from build123d import *

# Parameters (mm, degrees)
BOX005_W               = 0.7
BOX005_H               = 0.7
BOX005_DEPTH           = 6
BOX006_W               = 0.7
BOX006_H               = 0.7
BOX006_DEPTH           = 6
BOX007_W               = 0.7
BOX007_H               = 0.7
BOX007_DEPTH           = 6
BOX004_W               = 0.7
BOX004_H               = 0.7
BOX004_DEPTH           = 6
BOX009_W               = 10
BOX009_H               = 26
BOX009_DEPTH           = 2.7
BOX010_W               = 8.5
BOX010_H               = 15.8
BOX010_DEPTH           = 14
FILLET001_R            = 2
BOX008_W               = 10
BOX008_H               = 26
BOX008_DEPTH           = 2.7
CYLINDER001_R          = 1.6
CYLINDER001_DEPTH      = 8
CYLINDER002_R          = 1.6
CYLINDER002_DEPTH      = 8
CYLINDER003_R          = 1.6
CYLINDER003_DEPTH      = 8
CYLINDER004_R          = 1.6
CYLINDER004_DEPTH      = 8
CYLINDER005_R          = 1.6
CYLINDER005_DEPTH      = 8
CYLINDER006_R          = 1.6
CYLINDER006_DEPTH      = 8
CYLINDER007_R          = 1.6
CYLINDER007_DEPTH      = 8
CYLINDER_R             = 1.6
CYLINDER_DEPTH         = 8
BOX003_W               = 10
BOX003_H               = 10
BOX003_DEPTH           = 10
BOX003_ROLL_ANGLE      = 40.999967
BOX003_PLACEMENT_ANGLE = 180
BOX002_W               = 10
BOX002_H               = 10
BOX002_DEPTH           = 10
BOX002_ROLL_ANGLE      = 40.999967
BOX001_W               = 9.7
BOX001_H               = 17
BOX001_DEPTH           = 20.299999
FILLET_R               = 2


with BuildPart() as pin001:
    # Box005 → Box005 (new body)
    with BuildSketch(Plane(origin=(-5.35, 7.15, -3), x_dir=(1, 0, 0), z_dir=(0, 0, 1))):
        with Locations((0.35, 0.35)):
            Rectangle(BOX005_W, BOX005_H)
    extrude(amount=BOX005_DEPTH)


with BuildPart() as pin002:
    # Box006 → Box006 (new body)
    with BuildSketch(Plane(origin=(-5.35, -7.85, -3), x_dir=(1, 0, 0), z_dir=(0, 0, 1))):
        with Locations((0.35, 0.35)):
            Rectangle(BOX006_W, BOX006_H)
    extrude(amount=BOX006_DEPTH)


with BuildPart() as pin003:
    # Box007 → Box007 (new body)
    with BuildSketch(Plane(origin=(4.65, -7.85, -3), x_dir=(1, 0, 0), z_dir=(0, 0, 1))):
        with Locations((0.35, 0.35)):
            Rectangle(BOX007_W, BOX007_H)
    extrude(amount=BOX007_DEPTH)


with BuildPart() as pins:
    # Box004 → Box004 (new body)
    with BuildSketch(Plane(origin=(4.65, 7.15, -3), x_dir=(1, 0, 0), z_dir=(0, 0, 1))):
        with Locations((0.35, 0.35)):
            Rectangle(BOX004_W, BOX004_H)
    extrude(amount=BOX004_DEPTH)

    # Fusion003: union Pin001, Pin002, Pin003
    add(pin001.part)
    add(pin002.part)
    add(pin003.part)


with BuildPart() as box009:
    # Box009 → Box009 (new body)
    with BuildSketch(Plane(origin=(-2.25, 13, 0), x_dir=(-1, 0, 0), z_dir=(0, 0, 1))):
        with Locations((5, 13)):
            Rectangle(BOX009_W, BOX009_H)
    extrude(amount=BOX009_DEPTH)


with BuildPart() as fillet001:
    # Box010 → Box010 (new body)
    with BuildSketch(Plane(origin=(-4.25, -7.9, 0), x_dir=(1, 0, 0), z_dir=(0, 0, 1))):
        with Locations((4.25, 7.9)):
            Rectangle(BOX010_W, BOX010_H)
    extrude(amount=BOX010_DEPTH)

    # Fillet001
    fillet001_edges = [fillet001.edges().sort_by_distance(p)[0] for p in [
        (-4.25, -7.9, 7),
        (-4.25, 7.9, 7),
        (4.25, -7.9, 7),
        (4.25, 7.9, 7),
    ]]
    fillet(fillet001_edges, radius=FILLET001_R)


with BuildPart() as fusion004:
    # Box008 → Box008 (new body)
    with BuildSketch(Plane(origin=(2.25, -13, 0), x_dir=(1, 0, 0), z_dir=(0, 0, 1))):
        with Locations((5, 13)):
            Rectangle(BOX008_W, BOX008_H)
    extrude(amount=BOX008_DEPTH)

    # Fusion004: union Box009, Fillet001
    add(box009.part)
    add(fillet001.part)


with BuildPart() as cylinder001:
    # Cylinder001 → Cylinder001 (new body)
    with BuildSketch(Plane(origin=(-5, 2.5, 0), x_dir=(1, 0, 0), z_dir=(0, 0, 1))):
        Circle(CYLINDER001_R)
    extrude(amount=CYLINDER001_DEPTH)


with BuildPart() as cylinder002:
    # Cylinder002 → Cylinder002 (new body)
    with BuildSketch(Plane(origin=(-5, -2.5, 0), x_dir=(1, 0, 0), z_dir=(0, 0, 1))):
        Circle(CYLINDER002_R)
    extrude(amount=CYLINDER002_DEPTH)


with BuildPart() as cylinder003:
    # Cylinder003 → Cylinder003 (new body)
    with BuildSketch(Plane(origin=(-5, -7.5, 0), x_dir=(1, 0, 0), z_dir=(0, 0, 1))):
        Circle(CYLINDER003_R)
    extrude(amount=CYLINDER003_DEPTH)


with BuildPart() as cylinder004:
    # Cylinder004 → Cylinder004 (new body)
    with BuildSketch(Plane(origin=(5, 7.5, 0), x_dir=(1, 0, 0), z_dir=(0, 0, 1))):
        Circle(CYLINDER004_R)
    extrude(amount=CYLINDER004_DEPTH)


with BuildPart() as cylinder005:
    # Cylinder005 → Cylinder005 (new body)
    with BuildSketch(Plane(origin=(5, 2.5, 0), x_dir=(1, 0, 0), z_dir=(0, 0, 1))):
        Circle(CYLINDER005_R)
    extrude(amount=CYLINDER005_DEPTH)


with BuildPart() as cylinder006:
    # Cylinder006 → Cylinder006 (new body)
    with BuildSketch(Plane(origin=(5, -2.5, 0), x_dir=(1, 0, 0), z_dir=(0, 0, 1))):
        Circle(CYLINDER006_R)
    extrude(amount=CYLINDER006_DEPTH)


with BuildPart() as cylinder007:
    # Cylinder007 → Cylinder007 (new body)
    with BuildSketch(Plane(origin=(5, -7.5, 0), x_dir=(1, 0, 0), z_dir=(0, 0, 1))):
        Circle(CYLINDER007_R)
    extrude(amount=CYLINDER007_DEPTH)


with BuildPart() as pinholder:
    # Cylinder → Cylinder (new body)
    with BuildSketch(Plane(origin=(-5, 7.5, 0), x_dir=(1, 0, 0), z_dir=(0, 0, 1))):
        Circle(CYLINDER_R)
    extrude(amount=CYLINDER_DEPTH)

    # Fusion001: union Cylinder001, Cylinder002, Cylinder003, Cylinder004, Cylinder005, Cylinder006, Cylinder007
    add(cylinder001.part)
    add(cylinder002.part)
    add(cylinder003.part)
    add(cylinder004.part)
    add(cylinder005.part)
    add(cylinder006.part)
    add(cylinder007.part)


with BuildPart() as box003:
    # Box003 → Box003 (new body)
    with BuildSketch(Plane.XY):
        with Locations((5, 5)):
            Rectangle(BOX003_W, BOX003_H)
    extrude(amount=BOX003_DEPTH)


with BuildPart() as box003_1:
    # Box003 roll: moved
    add(box003.part.rotate(Axis((0, 0, 0), (1, 0, 0)), BOX003_ROLL_ANGLE))


with BuildPart() as box003_2:
    # Box003 placement: moved
    add(box003_1.part.moved(Location((10, -0.7, 14))).rotate(Axis((10, -0.7, 14), (0, 0, 1)), BOX003_PLACEMENT_ANGLE))


with BuildPart() as fusion:
    # Box002 → Box002 (new body)
    with BuildSketch(Plane.XY):
        with Locations((5, 5)):
            Rectangle(BOX002_W, BOX002_H)
    extrude(amount=BOX002_DEPTH)


with BuildPart() as fusion_1:
    # Box002 roll: moved
    add(fusion.part.rotate(Axis((0, 0, 0), (1, 0, 0)), BOX002_ROLL_ANGLE))


with BuildPart() as fusion_2:
    # Box002 placement: moved
    add(fusion_1.part.moved(Location((0, 17.7, 14))))

    # Fusion: union Box003
    add(box003_2.part)


with BuildPart() as obj1:
    # Box001 → Box001 (new body)
    with BuildSketch(Plane.XY):
        with Locations((4.85, 8.5)):
            Rectangle(BOX001_W, BOX001_H)
    extrude(amount=BOX001_DEPTH)

    # Cut: cut Fusion
    add(fusion_2.part, mode=Mode.SUBTRACT)

    # Fillet
    fillet_edges = [obj1.edges().sort_by_distance(p)[0] for p in [
        (0, 0, 7.402629),
        (0, 2.38825, 17.552629),
        (0, 14.61175, 17.552629),
        (0, 17, 7.402629),
        (9.7, 17, 7.402629),
        (9.7, 0, 7.402629),
        (9.7, 2.38825, 17.552629),
        (9.7, 14.61175, 17.552629),
    ]]
    fillet(fillet_edges, radius=FILLET_R)


with BuildPart() as obj1_1:
    # Fillet placement: moved
    add(obj1.part.moved(Location((-4.85, -8.5, 0))))

    # Fusion002: union pinholder
    add(pinholder.part)

    # Cut001: cut Fusion004
    add(fusion004.part, mode=Mode.SUBTRACT)

    # Fusion005: union Pins
    add(pins.part)


solid = obj1_1.part
Model file for the job. Use its own axes, mm. A direction names the side the tool comes from. Coordinates: 2 decimals unless noted, no trailing zeros. Order: outer loops, then holes, each group sorted by start corner. A loop starts at its lowest first (then second) coordinate and runs counter-clockwise, first axis right, second up. Notation, with made-up numbers: (68.25, 5.25) -> (105.25, 5.25) arc R35 cw to (105.25, 41.25) -> close; hole circle Ø4 at (42, 13.25). An arc over 180 degrees is marked (long way). Return JSON: item names as keys, results as strings. Group by question number.
Item 1: Saw through at A-A on z = 13.25. Write the cut outline in (x, y).
Item 2: Wall check: line 1 along Y through (x, z) = (1.25, 8.5); line 2 along X through (y, z) = (-0.5, 11.5); line 3 along Y through (x, z) = (5.25, 3.5). Give the ranges that are in metal, low to high. Write a range as [from, to].
Item 3: Saw through at B-B on y = 0. Write the cut outline in (x, z).
Item 4: Saw through at C-C on x = 0. Write the cut outline in (y, z), then the cut area to 3 significant figures.
Item 5: Tool access for faces 4 (the flat face through (6, 3, 8)), 5 (the flat face through (0, 0, 14)), 6 (the flat face through (-6, -2, 8)), 7 (the flat face through (0, 8.5, 7)), 8 (the cylindrical face through (-4.015, -8.126, 10.182)): list every direction of +Z, -Z, +X, -X, +Y, -Y with a clear straight run to the whole face (end or side of a thin tool).
Item 6: Pull direction Y, two halves, no side cores. Call faces 1 (the cylindrical face through (4.249, -5.727, 17.126)), 2 (the flat face through (6, -2, 8)), 3 (the cylindrical face through (-3.68, 7.3, 8.43)): pulls with the +Y half, pulls with the -Y half, needs draft (parallel to the pull), parting line crosses it, or undercut.
Item 7: Flat gauge pins, fed straight in: P1, Ø1.5, axis at y = 3.5, z = 3, coming from the +X side; P2, Ø0.9, axis at x = 5.5, y = -8, coming from the +Z side; P3, Ø0.6, axis at y = 7.5, z = 1, coming from the +X side. Where does each tip first touch, or does it go through?
Values found:
{
 "1": {"outline": "(-4.85, -6.5) arc R2 ccw to (-2.85, -8.5) -> (2.85, -8.5) arc R2 ccw to (4.85, -6.5) -> (4.85, 6.5) arc R2 ccw to (2.85, 8.5) -> (-2.85, 8.5) arc R2 ccw to (-4.85, 6.5) -> close; hole (-4.25, -5.9) arc R2 ccw to (-2.25, -7.9) -> (2.25, -7.9) arc R2 ccw to (4.25, -5.9) -> (4.25, 5.9) arc R2 ccw to (2.25, 7.9) -> (-2.25, 7.9) arc R2 ccw to (-4.25, 5.9) -> close"},
 "2": {"line 1": "y = [-8.5, -7.9], [7.9, 8.5]", "line 2": "x = [-4.85, -4.25], [4.25, 4.85]", "line 3": "y = [-9.08, -5.92], [-4.08, -0.92], [0.92, 4.08], [5.92, 9.08]"},
 "3": {"outline": "(-4.85, 2.7) -> (-4.25, 2.7) -> (-4.25, 14) -> (4.25, 14) -> (4.25, 2.7) -> (4.85, 2.7) -> (4.85, 20.3) -> (-4.85, 20.3) -> close"},
 "4": {"outline": "(-8.5, 0) -> (-7.9, 0) -> (-7.9, 14) -> (7.9, 14) -> (7.9, 0) -> (8.5, 0) -> (8.5, 14.81) -> (3.72, 20.3) -> (-3.72, 20.3) -> (-8.5, 14.81) -> close", "area": "97.7 mm2"},
 "5": {"face 4": "+Z, +X, +Y, -Y", "face 5": "-Z", "face 6": "+Z, -X, +Y, -Y", "face 7": "+Z, -Z, +Y", "face 8": "+Z, -Y"},
 "6": {"face 1": "pulls with the -Y half", "face 2": "needs draft", "face 3": "undercut"},
 "7": {"P1": "stops at x = 6.58", "P2": "stops at z = 8", "P3": "stops at x = 5.35"}
}
